Read the model definition and answer for the solid it produces. Units are mm, in the model's axes. A direction names the side the tool comes from. Coordinates: 2 decimals unless noted, no trailing zeros. Order: outer loops, then holes, each group sorted by start corner. A loop starts at its lowest first (then second) coordinate and runs counter-clockwise, first axis right, second up. Notation, with made-up numbers: (80.25, -6) -> (110.25, -6) arc R14 cw to (110.25, 11) -> close; hole circle Ø10 at (12, -32). An arc over 180 degrees is marked (long way). Answer as a JSON object with one key per item and string values. Group by question number.
1) Section C-C on y = -13 is taken. Determine the outline of the cut face in (x, z).
2) Section D-D on x = -10.25 is taken. Determine the outline of the cut face in (y, z), and give its area (3 significant figures).
3) A tool of negligible diameter and unlimited length cuts with its end or side. For faces 1 (the flat face through (0, -1, -12)), 2 (the flat face through (-2, -1, -2)), from which of +Z, -Z, +X, -X, +Y, -Y can it reach the whole face along a straight path? Write none if from no direction.
4) Determine the mould class of faces 3 (the cylindrical face through (-0.03, 43.26, -2.61)), 4 (the flat face through (-7, 1, 8)), 5 (the flat face through (-1.8, 52.5, 2.5)), 6 (the flat face through (-5, 1, 12)) for opening direction Z: released by +Z, released by -Z, zero draft, split by the parting line, or undercut.
5) Section A-A on z = -4.25 is taken. Determine the outline of the cut face in (x, y), and give its area (3 significant figures).
6) Section B-B on y = 40 is taken. Determine the outline of the cut face in (x, z), and give its area (3 significant figures).
7) Given pin 1 (2 mm diameter, centred on x = -4.5, y = 33, fed in from -Z); pin 2 (12 mm diameter, centred on y = 19.5, z = -5.5, fed in from -X), each flat-ended and moving along its own axis, determine where each tip first touches the part or whether it passes through.
8) Consider L1, parallel to Z at x = -6, y = 10; L2, parallel to X at y = 0, z = -9.25; L3, parallel to Y at x = -0.75, z = 1.5. Determine where each line is inside the solid, lowest interval first.
from build123d import *

# Parameters (mm, degrees)
F0_W          = 105
F0_H          = 24
F1_DEPTH      = 2
F1_DEPTH_BACK = 2
F2_W          = 105
F2_H          = 4
F3_DEPTH      = 10
F4_R          = 5.320603
F5_DEPTH      = 4.001


with BuildPart() as f1:
    # F0 (on Right) → F1 (new body, two sides)
    with BuildSketch(Plane.YZ) as f1_sk:
        Rectangle(F0_W, F0_H)
    extrude(amount=F1_DEPTH)
    extrude(f1_sk.sketch, amount=-F1_DEPTH_BACK)

    # F2 (on face) → F3 (join)
    with BuildSketch(Plane(origin=(-2, 0, 0), x_dir=(0, -1, 0), z_dir=(-1, 0, 0))):
        with Locations((0, 10)):
            Rectangle(F2_W, F2_H)
    extrude(amount=F3_DEPTH)

    # F4 (on face) → F5 (cut, through all)
    with BuildSketch(Plane(origin=(-2, 0, 0), x_dir=(0, -1, 0), z_dir=(-1, 0, 0))):
        with Locations((-37.945189, -2.843227)):
            Circle(F4_R)
    extrude(amount=-F5_DEPTH, mode=Mode.SUBTRACT)


solid = f1.part
Worked answers:
{
 "1": {"outline": "(-12, 8) -> (-2, 8) -> (-2, -12) -> (2, -12) -> (2, 12) -> (-12, 12) -> close"},
 "2": {"outline": "(-52.5, 8) -> (52.5, 8) -> (52.5, 12) -> (-52.5, 12) -> close", "area": "420 mm²"},
 "3": {"face 1": "-Z, +X, -X, +Y, -Y", "face 2": "-Z, -X, +Y, -Y"},
 "4": {"face 3": "undercut", "face 4": "released by -Z", "face 5": "zero draft", "face 6": "released by +Z"},
 "5": {"outline": "(-2, -52.5) -> (2, -52.5) -> (2, 32.81) -> (-2, 32.81) -> close; (-2, 43.08) -> (2, 43.08) -> (2, 52.5) -> (-2, 52.5) -> close", "area": "379 mm²"},
 "6": {"outline": "(-12, 8) -> (-2, 8) -> (-2, 2.06) -> (2, 2.06) -> (2, 12) -> (-12, 12) -> close; (-2, -12) -> (2, -12) -> (2, -7.75) -> (-2, -7.75) -> close", "area": "96.7 mm²"},
 "7": {"pin 1": "stops at z = 8", "pin 2": "stops at x = -2"},
 "8": {"L1": "z = 8 to 12", "L2": "x = -2 to 2", "L3": "y = -52.5 to 34.87, 41.02 to 52.5"}
}
